```python
from build123d import *

# Parameters (mm, degrees)
SKETCH11_R          = 35
BOSS_EXTRUDE2_DEPTH = 263.365760626
FILLET2_R           = 10
SKETCH15_R          = 20
CUT_EXTRUDE1_DEPTH  = 271.0000001


with BuildPart() as part:
    # Sketch14 → Revolve3 (revolve)
    with BuildSketch(Plane.XY):
        Polygon((30, -115), (30, 135), (20, 135), (20, -135), (50, -135), (50, -115), align=None)
    revolve(axis=Axis((0, -135, 0), (0, 1, 0)))

    # Sketch11 → Boss-Extrude2 (add)
    with BuildSketch(Plane(origin=(0.069700253, 0.395289776, -0.070775492), x_dir=(-0.03015369, -0.171010072, -0.984807753), z_dir=(0.984807753, -0.173648178, 0))):
        with Locations((-5.721541908, 32.04089679)):
            Circle(SKETCH11_R)
    extrude(amount=-BOSS_EXTRUDE2_DEPTH)

    # Fillet2
    fillet2_edges = [part.edges().sort_by_distance(p)[0] for p in [
        (-30, -115, 0),
    ]]
    fillet(fillet2_edges, radius=FILLET2_R)

    # Sketch15 → Cut-Extrude1 (cut, through all)
    with BuildSketch(Plane(origin=(0, 135, 0), x_dir=(1, 0, 0), z_dir=(0, 1, 0))):
        Circle(SKETCH15_R)
    extrude(amount=-CUT_EXTRUDE1_DEPTH, mode=Mode.SUBTRACT)


solid = part.part
```
Source: CAD feature listing. Evaluate the final solid. Frame: model axes, mm. A direction names the side the tool comes from. Give positions to 0.01 mm unless a question says otherwise; leave off trailing zeros. Loops run counter-clockwise (first coordinate to the right, second up) from the corner with the lowest first, then second, coordinate; pieces in that order, holes last. Notation, with made-up numbers: (86, 13.5) -> (119, 13.5) arc R34 cw to (119, 46.5) -> close; hole circle Ø8 at (21, -8.75). An arc over 180 degrees is marked (long way). Use a Markdown table: item, result. Add a question column.
(1) Section query B-B (y = -57). Output: boundary loops of the cut face in (x, z), then the cut area to 3 significant figures.
(2) Section query A-A (z = 0). Output: boundary loops of the cut face in (x, y), then the cut area to 3 significant figures.
(3) Access query for faces 4 (the face through (5.876, 33.322, -31.512)), 5 (the face through (28.615, 16.68, -9.011)), 6 (the face through (1, -135, 22)). Directions: +Z, -Z, +X, -X, +Y, -Y. A direction counts if a zero-diameter tool reaches every point of the face in a straight line with its end or side. Return the directions, or none.
(4) First-contact query: pin 1 Ø3 at (y, z) = (-27.5, 4.5) entering from -X; pin 2 Ø4 at (x, z) = (-125, 32) entering from -Y; pin 3 Ø4 at (y, z) = (108, -12) entering from -X. Flat tips, straight axial feed; report the tip coordinate or a pass-through.
(5) Ray query, line 1 (Z direction, x = 0, y = -52); line 2 (X direction, y = -75, z = 4). Return the intervals inside material, ascending.
(6) Pull-direction query (X, two-part tool) for faces 1 (the face through (6.027, 34.181, 31.846)), 2 (the face through (-4.336, -1.89, 19.524)), 3 (the face through (47.69, -124.86, -15.02)); classes: +X half, -X half, draft (parallel to the pull), parting line (faces both ways), or undercut.
Checked values:
| question | item | result |
|---|---|---|
| 1 | outline | circle Ø60 at (0, 0); hole circle Ø40 at (0, 0) |
| 1 | area | 1,570 mm^2 |
| 2 | outline | (-259.72, 43.71) -> (-30, 3.21) -> (-30, -105) arc R10 cw to (-40, -115) -> (-50, -115) -> (-50, -135) -> (-20, -135) -> (-20, 135) -> (-30, 135) -> (-30, 74.29) -> (-247.57, 112.65) -> close; (20, -135) -> (50, -135) -> (50, -115) -> (40, -115) arc R10 cw to (30, -105) -> (30, 135) -> (20, 135) -> close |
| 2 | area | 22,100 mm^2 |
| 3 | face 4 | -Z, +X |
| 3 | face 5 | none |
| 3 | face 6 | +Z, -Z, +X, -X, -Y |
| 4 | pin 1 | x = -29.85 |
| 4 | pin 2 | y = 37.17 |
| 4 | pin 3 | x = -248.74 |
| 5 | line 1 | -30 to -20, 20 to 30 |
| 5 | line 2 | -29.73 to -19.6, 19.6 to 29.73 |
| 6 | face 1 | +X half |
| 6 | face 2 | undercut |
| 6 | face 3 | parting line |
